The listing builds one solid part. Answer for the finished solid, in the listing's coordinates (mm). Round coordinates to 2 decimals unless told otherwise and drop trailing zeros. Write each loop counter-clockwise with the first axis right and the second up, starting at its lowest first coordinate (ties: lowest second). Pieces come first, ordered by that corner, then holes.
Item 1: Find the intervals of material crossed by probe 1 along Z at (x, y) = (38.1, 1.9); probe 2 along X at (y, z) = (1.7, -17), in increasing order.
Item 2: Find section B-B on x = 38.1. Give the vertices of the cut face in (y, z) (3 decimals).
Item 3: Find section A-A on z = -19.05. Give the vertices of the cut face in (x, y) (3 decimals), then the cut area to 3 significant figures.
Item 4: Find section C-C on y = 2.35. Give the number of separate pieces and of enclosed holes in the cut face, then the cut area to 3 significant figures.
Item 5: Find section D-D on x = -79.5. Give the vertices of the cut face in (y, z) (3 decimals), then the cut area to 3 significant figures.
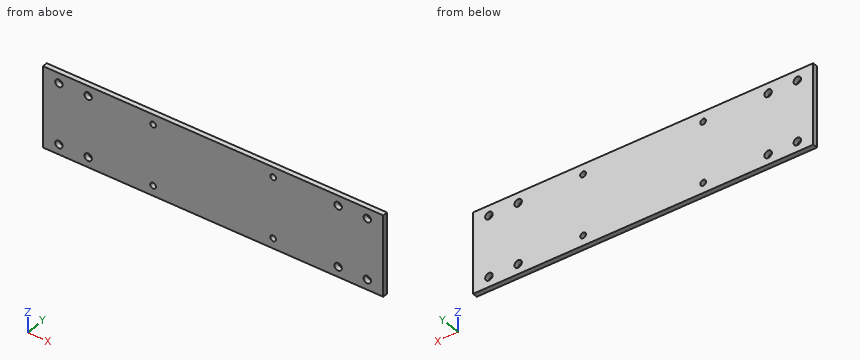
```python
from build123d import *

# Parameters (mm, degrees)
SKETCH1_W           = 215.9
SKETCH1_H           = 50.8
SKETCH1_R           = 1.80975
BOSS_EXTRUDE1_DEPTH = 3.175
SKETCH2_R           = 2.3495
CUT_EXTRUDE1_DEPTH  = 4.175


with BuildPart() as part:
    # Sketch1 → Boss-Extrude1 (new body)
    with BuildSketch(Plane(origin=(0, 0, 0), x_dir=(1, 0, 0), z_dir=(0, 1, 0))):
        Rectangle(SKETCH1_W, SKETCH1_H)
        with Locations((-38.1, 19.05)):
            Circle(SKETCH1_R, mode=Mode.SUBTRACT)
        with Locations((-38.1, -19.05)):
            Circle(SKETCH1_R, mode=Mode.SUBTRACT)
        with Locations((38.1, 19.05)):
            Circle(SKETCH1_R, mode=Mode.SUBTRACT)
        with Locations((38.1, -19.05)):
            Circle(SKETCH1_R, mode=Mode.SUBTRACT)
    extrude(amount=BOSS_EXTRUDE1_DEPTH)

    # Sketch2 → Cut-Extrude1 (cut, through all)
    with BuildSketch(Plane(origin=(0, 3.175, 0), x_dir=(1, 0, 0), z_dir=(0, 1, 0))):
        with Locations((-97.8535, 19.05)):
            Circle(SKETCH2_R)
        with Locations((-79.3115, 19.05)):
            Circle(SKETCH2_R)
        with Locations((-79.3115, -19.05)):
            Circle(SKETCH2_R)
        with Locations((-97.8535, -19.05)):
            Circle(SKETCH2_R)
        with Locations((97.8535, -19.05)):
            Circle(SKETCH2_R)
        with Locations((79.3115, -19.05)):
            Circle(SKETCH2_R)
        with Locations((79.3115, 19.05)):
            Circle(SKETCH2_R)
        with Locations((97.8535, 19.05)):
            Circle(SKETCH2_R)
    extrude(amount=-CUT_EXTRUDE1_DEPTH, mode=Mode.SUBTRACT)


solid = part.part
```
Check values:
1. probe 1: z = -25.4 to -20.86, -17.24 to 17.24, 20.86 to 25.4
1. probe 2: x = -107.95 to -99, -96.71 to -80.46, -78.16 to 78.16, 80.46 to 96.71, 99 to 107.95
2. outline: (0, -25.4) - (3.175, -25.4) - (3.175, -20.86) - (0, -20.86) - close; (0, -17.24) - (3.175, -17.24) - (3.175, 17.24) - (0, 17.24) - close; (0, 20.86) - (3.175, 20.86) - (3.175, 25.4) - (0, 25.4) - close
3. outline: (-107.95, 0) - (-100.203, 0) - (-100.203, 3.175) - (-107.95, 3.175) - close; (-95.504, 0) - (-81.661, 0) - (-81.661, 3.175) - (-95.504, 3.175) - close; (-76.962, 0) - (-39.91, 0) - (-39.91, 3.175) - (-76.962, 3.175) - close; (-36.29, 0) - (36.29, 0) - (36.29, 3.175) - (-36.29, 3.175) - close; (39.91, 0) - (76.962, 0) - (76.962, 3.175) - (39.91, 3.175) - close; (81.661, 0) - (95.504, 0) - (95.504, 3.175) - (81.661, 3.175) - close; (100.203, 0) - (107.95, 0) - (107.95, 3.175) - (100.203, 3.175) - close
3. area: 603 mm2
4. separate pieces: 1
4. enclosed holes: 12
4. area: 10,800 mm2
5. outline: (0, -25.4) - (3.175, -25.4) - (3.175, -21.392) - (0, -21.392) - close; (0, -16.708) - (3.175, -16.708) - (3.175, 16.708) - (0, 16.708) - close; (0, 21.392) - (3.175, 21.392) - (3.175, 25.4) - (0, 25.4) - close
5. area: 132 mm2
